Autodesk Fusion 360 part; units mm, degrees
sketch "Sketch1" plane through (0, 0, 0) normal (0, 1, 0) x (1, 0, 0)
  line L0 (35.25, -35.25) -> (-35.25, -35.25)
  line L1 (-35.25, -35.25) -> (-35.25, 35.25)
  line L2 (-35.25, 35.25) -> (35.25, 35.25)
  line L3 (35.25, 35.25) -> (35.25, -35.25)
  line L4 (35.25, -35.25) -> (-35.25, 35.25) construction
  line L5 (-35.25, -35.25) -> (35.25, 35.25) construction
  dimension "d1" = 70.5
  dimension "d2" = 70.5
extrude "Extrude1" add sketch "Sketch1" along normal blind 2
fillet "Fillet1" radius 6.75 4 edges at (-35.25, 1, 35.25) (-35.25, 1, -35.25) (35.25, 1, 35.25) (35.25, 1, -35.25)
fillet "Fillet2" radius 2 8 edges at (0, 0, -35.25) (-33.273, 0, -33.273) (-35.25, 0, 0) (-33.273, 0, 33.273) (0, 0, 35.25) (33.273, 0, 33.273) (35.25, 0, 0) (33.273, 0, -33.273)
extrude "Extrude2" add 1 faces at (9.5, 2, 11.75) along direction (0, 1, 0) blind 1
The listing builds one solid part. Answer for the finished solid, in the listing's coordinates (mm). Round coordinates to 2 decimals unless told otherwise and drop trailing zeros. Order: outer loops, then holes, each group sorted by start corner. A loop starts at its lowest first (then second) coordinate and runs counter-clockwise, first axis right, second up. Notation, with made-up numbers: M 37.25,53 L 46.25,53 A36 ccw 46.25,89 Z; hole C -2.75,3.25 d9. An arc over 180 degrees is marked long. Answer in a Markdown table with one row per item. Add a question column.
1) Consider line 1 along X through (y, z) = (1.75, 18.5); line 2 along Z through (x, y) = (-26, 0.45); line 3 along Z through (x, y) = (1, 1). Determine where each line is inside the solid, lowest interval first. Write a range as from..to.
2) A flat-ended cylindrical pin translates along its axis: pin 1 Ø1.5 at (x, y) = (21.5, 1) entering from +Z. Find the tip coordinate at first contact, or state that the pin passes through.
3) The part is cut by section A-A on y = 1.05. Determine the outline of the cut face in (x, z).
Findings below:
| question | item | result |
|---|---|---|
| 1 | line 1 | x = -35.23..35.23 |
| 1 | line 2 | z = -34.51..34.51 |
| 1 | line 3 | z = -34.98..34.98 |
| 2 | pin 1 | stops at z = 35.23 |
| 3 | outline | M -35.01,-28.5 A6.51 ccw -28.5,-35.01 L 28.5,-35.01 A6.51 ccw 35.01,-28.5 L 35.01,28.5 A6.51 ccw 28.5,35.01 L -28.5,35.01 A6.51 ccw -35.01,28.5 Z |
